Read the model definition and answer for the solid it produces. Units are mm, in the model's axes. A direction names the side the tool comes from. Give positions to 0.01 mm unless a question says otherwise; leave off trailing zeros. Order: outer loops, then holes, each group sorted by start corner. A loop starts at its lowest first (then second) coordinate and runs counter-clockwise, first axis right, second up. Notation, with made-up numbers: (82.5, 51.25) - (133.5, 51.25) arc R16 cw to (133.5, 63.25) - close; hole circle Ø10 at (79.5, 2). An arc over 180 degrees is marked (long way). Return JSON: item names as keys, results as strings.
```python
from build123d import *

# Parameters (mm, degrees)
ESBO_O1_W                = 67
ESBO_O1_H                = 33
ESBO_O1_W_2              = 60.7
ESBO_O1_H_2              = 26.7
ESBO_O1_W_3              = 12.2
RESSALTO_EXTRUS_O4_DEPTH = 20
ESBO_O3_W                = 48.5
ESBO_O3_H                = 26.7
RESSALTO_EXTRUS_O5_DEPTH = 2
RESSALTO_EXTRUS_O9_START = 18.15
ESBO_O4_R                = 3.9
ESBO_O4_R_2              = 2.83
RESSALTO_EXTRUS_O9_DEPTH = 2


with BuildPart() as part:
    # Esboço1 → Ressalto-extrusão4 (new body)
    # profile 1 of 2: a face of its own
    with BuildSketch(Plane(origin=(0, 0, 0), x_dir=(1, 0, 0), z_dir=(0, 1, 0))):
        Rectangle(ESBO_O1_W, ESBO_O1_H)
        Rectangle(ESBO_O1_W_2, ESBO_O1_H_2, mode=Mode.SUBTRACT)
    # profile 2 of 2: a face of its own
    with BuildSketch(Plane(origin=(0, 0, 0), x_dir=(1, 0, 0), z_dir=(0, 1, 0))):
        with Locations((24.25, 0)):
            Rectangle(ESBO_O1_W_3, ESBO_O1_H_2)
    extrude(amount=RESSALTO_EXTRUS_O4_DEPTH)

    # Esboço3 → Ressalto-extrusão5 (add)
    with BuildSketch(Plane(origin=(0, 0, 0), x_dir=(1, 0, 0), z_dir=(0, 1, 0))):
        with Locations((-6.1, 0)):
            Rectangle(ESBO_O3_W, ESBO_O3_H)
    extrude(amount=RESSALTO_EXTRUS_O5_DEPTH)

    # Esboço4 → Ressalto-extrusão9 (add)
    # profile 1 of 2: a face of its own
    with BuildSketch(Plane(origin=(0, 0, 0), x_dir=(0, 0, -1), z_dir=(1, 0, 0)).offset(RESSALTO_EXTRUS_O9_START)):
        with Locations((6.35, 10.75)):
            Circle(ESBO_O4_R)
        with Locations((6.35, 10.75)):
            Circle(ESBO_O4_R_2, mode=Mode.SUBTRACT)
    # profile 2 of 2: a face of its own
    with BuildSketch(Plane(origin=(0, 0, 0), x_dir=(0, 0, -1), z_dir=(1, 0, 0)).offset(RESSALTO_EXTRUS_O9_START)):
        with Locations((-6.35, 10.75)):
            Circle(ESBO_O4_R_2)
    extrude(amount=-RESSALTO_EXTRUS_O9_DEPTH)


solid = part.part
```
Q1. Consider L1, parallel to Y at x = 16.95, z = -6.35; L2, parallel to X at y = 8, z = -4; L3, parallel to X at y = 7, z = 1.5. Determine where each line is inside the solid, lowest interval first.
Values:
{"L1": "y = 0 to 2, 6.85 to 7.92, 13.58 to 14.65", "L2": "x = -33.5 to -30.35, 16.15 to 33.5", "L3": "x = -33.5 to -30.35, 18.15 to 33.5"}
Q2. For faces 4 (the flat face through (-33.5, 10, 0)), 5 (the flat face through (-6, 11, 13.35)), 6 (the cylindrical face through (17.164, 7.987, 6.963)), determine the directions among +Z, -Z, +X, -X, +Y, -Y from which every point of the face is accessible in a straight line to the end or side of a thin tool.
Values:
{"face 4": "+Z, -Z, -X, +Y, -Y", "face 5": "+Y", "face 6": "none"}
Q3. Given pin 1 (13.5 mm diameter, centred on x = -3.5, z = 3, fed in from +Y), flat-ended and moving along its own axis, determine where the tip first touches the part or whether it passes through.
Values:
{"pin 1": "stops at y = 2"}
Q4. A cutting plane is placed at D-D (z = -6.35). Write down the section's boundary in (x, y).
Values:
{"outline": "(-33.5, 0) - (33.5, 0) - (33.5, 20) - (18.15, 20) - (18.15, 14.65) - (16.15, 14.65) - (16.15, 13.58) - (18.15, 13.58) - (18.15, 7.92) - (16.15, 7.92) - (16.15, 6.85) - (18.15, 6.85) - (18.15, 2) - (-30.35, 2) - (-30.35, 20) - (-33.5, 20) - close"}
Q5. Determine the mould class of faces 1 (the flat face through (-30.35, 11, 0)), 2 (the cylindrical face through (17.164, 7.987, -5.737)), 3 (the flat face through (22, 20, 0)) for opening direction Y: released by +Y, released by -Y, zero draft, split by the parting line, or undercut.
Values:
{"face 1": "zero draft", "face 2": "undercut", "face 3": "released by +Y"}
Q6. A cutting plane is placed at B-B (z = 6.35). Write down the section's boundary in (x, y).
Values:
{"outline": "(-33.5, 0) - (33.5, 0) - (33.5, 20) - (18.15, 20) - (18.15, 13.58) - (16.15, 13.58) - (16.15, 7.92) - (18.15, 7.92) - (18.15, 2) - (-30.35, 2) - (-30.35, 20) - (-33.5, 20) - close"}
Q7. A cutting plane is placed at C-C (x = -7). Write down the section's boundary in (y, z).
Values:
{"outline": "(0, -16.5) - (20, -16.5) - (20, -13.35) - (2, -13.35) - (2, 13.35) - (20, 13.35) - (20, 16.5) - (0, 16.5) - close"}
Q8. A cutting plane is placed at A-A (y = 10.75). Write down the section's boundary in (x, z), and give its area (3 significant figures).
Values:
{"outline": "(-33.5, -16.5) - (33.5, -16.5) - (33.5, 16.5) - (-33.5, 16.5) - close; hole (-30.35, -13.35) - (18.15, -13.35) - (18.15, -10.25) - (16.15, -10.25) - (16.15, -9.18) - (18.15, -9.18) - (18.15, -3.52) - (16.15, -3.52) - (16.15, -2.45) - (18.15, -2.45) - (18.15, 3.52) - (16.15, 3.52) - (16.15, 9.18) - (18.15, 9.18) - (18.15, 13.35) - (-30.35, 13.35) - close", "area": "932 mm²"}
